from build123d import *

# Parameters (mm, degrees)
SKETCH1_W              = 144.4879
SKETCH1_H              = 47.625
SKETCH1_R              = 14.3129
BOSS_EXTRUDE1_DEPTH    = 6.35
FILLET1_R              = 6.35
F_10_32_TAPPED_HOLE1_D = 4.0386
F_10_32_TAPPED_HOLE2_D = 4.0386
CUT_EXTRUDE1_DEPTH     = 147.5745916
FILLET2_R              = 2.54


with BuildPart() as part:
    # Sketch1 → Boss-Extrude1 (new body)
    with BuildSketch(Plane(origin=(0, 0, 0), x_dir=(0, 0, -1), z_dir=(1, 0, 0))):
        with Locations((-72.24395, 0)):
            Rectangle(SKETCH1_W, SKETCH1_H)
        with Locations((-120.65, 0)):
            Circle(SKETCH1_R, mode=Mode.SUBTRACT)
    extrude(amount=BOSS_EXTRUDE1_DEPTH)

    # Fillet1
    fillet1_edges = [part.edges().sort_by_distance(p)[0] for p in [
        (3.175, -23.8125, 144.4879),
        (3.175, 23.8125, 144.4879),
        (3.175, 23.8125, 0),
        (3.175, -23.8125, 0),
    ]]
    fillet(fillet1_edges, radius=FILLET1_R)

    # #10-32 Tapped Hole1 (through all)
    with Locations(Plane.ZY):
        with Locations((103.1875, 17.4625), (138.1125, 17.4625), (138.1125, -17.4625), (103.1875, -17.4625)):
            Hole(F_10_32_TAPPED_HOLE1_D / 2)

    # #10-32 Tapped Hole2 (through all)
    with Locations(Plane(origin=(6.35, 0, 0), x_dir=(0, 0, -1), z_dir=(1, 0, 0))):
        with Locations((-12.7, 14.2875), (-38.1, 14.2875), (-38.1, -11.1125), (-12.7, -11.1125)):
            Hole(F_10_32_TAPPED_HOLE2_D / 2)

    # Sketch8 → Cut-Extrude1 (cut, through all)
    with BuildSketch(Plane(origin=(6.35, 0, 0), x_dir=(0, 0, -1), z_dir=(1, 0, 0))):
        with BuildLine():
            Line((-80.436721657, 17.4625), (-53.975, 17.4625))
            ThreePointArc((-53.975, 17.4625), (-51.72993597, 16.53256403), (-50.8, 14.2875))
            Line((-50.8, 14.2875), (-50.8, -5.989274253))
            ThreePointArc((-50.8, -5.989274253), (-52.569784121, -8.836376874), (-55.906137534, -8.509459331))
            Line((-55.906137534, -8.509459331), (-82.367859191, 11.767314922))
            ThreePointArc((-82.367859191, 11.767314922), (-83.443564904, 15.307067893), (-80.436721657, 17.4625))
        make_face()
        with BuildLine():
            Line((-93.6625, 5.989274253), (-93.6625, -14.2875))
            ThreePointArc((-93.6625, -14.2875), (-92.73256403, -16.53256403), (-90.4875, -17.4625))
            Line((-90.4875, -17.4625), (-64.025778343, -17.4625))
            ThreePointArc((-64.025778343, -17.4625), (-61.018935096, -15.307067893), (-62.094640809, -11.767314922))
            Line((-62.094640809, -11.767314922), (-88.556362466, 8.509459331))
            ThreePointArc((-88.556362466, 8.509459331), (-91.892715879, 8.836376874), (-93.6625, 5.989274253))
        make_face()
        with BuildLine():
            Line((-38.1, 19.05), (-12.7, 19.05))
            ThreePointArc((-12.7, 19.05), (-16.728416874, 16.827827486), (-16.997532015, 12.235032015))
            Line((-16.997532015, 12.235032015), (-25.4, 3.83256403))
            Line((-25.4, 3.83256403), (-33.802467985, 12.235032015))
            ThreePointArc((-33.802467985, 12.235032015), (-34.071583126, 16.827827486), (-38.1, 19.05))
        make_face()
        with BuildLine():
            Line((-7.9375, 14.2875), (-7.9375, -11.1125))
            ThreePointArc((-7.9375, -11.1125), (-10.159672514, -7.084083126), (-14.752467985, -6.814967985))
            Line((-14.752467985, -6.814967985), (-23.15493597, 1.5875))
            Line((-23.15493597, 1.5875), (-14.752467985, 9.989967985))
            ThreePointArc((-14.752467985, 9.989967985), (-10.159672514, 10.259083126), (-7.9375, 14.2875))
        make_face()
        with BuildLine():
            Line((-38.1, -15.875), (-12.7, -15.875))
            ThreePointArc((-12.7, -15.875), (-16.728416874, -13.652827486), (-16.997532015, -9.060032015))
            Line((-16.997532015, -9.060032015), (-25.4, -0.65756403))
            Line((-25.4, -0.65756403), (-33.802467985, -9.060032015))
            ThreePointArc((-33.802467985, -9.060032015), (-34.071583126, -13.652827486), (-38.1, -15.875))
        make_face()
        with BuildLine():
            Line((-42.8625, 14.2875), (-42.8625, -11.1125))
            ThreePointArc((-42.8625, -11.1125), (-40.640327486, -7.084083126), (-36.047532015, -6.814967985))
            Line((-36.047532015, -6.814967985), (-27.64506403, 1.5875))
            Line((-27.64506403, 1.5875), (-36.047532015, 9.989967985))
            ThreePointArc((-36.047532015, 9.989967985), (-40.640327486, 10.259083126), (-42.8625, 14.2875))
        make_face()
    extrude(amount=-CUT_EXTRUDE1_DEPTH, mode=Mode.SUBTRACT)

    # Fillet2
    fillet2_edges = [part.edges().sort_by_distance(p)[0] for p in [
        (3.175, -15.875, 12.7),
    ]]
    fillet(fillet2_edges, radius=FILLET2_R)
    fillet2_2_edges = [part.edges().sort_by_distance(p)[0] for p in [
        (3.175, -9.060032015, 16.997532015),
    ]]
    fillet(fillet2_2_edges, radius=FILLET2_R)
    fillet2_3_edges = [part.edges().sort_by_distance(p)[0] for p in [
        (3.175, -0.65756403, 25.4),
    ]]
    fillet(fillet2_3_edges, radius=FILLET2_R)
    fillet2_4_edges = [part.edges().sort_by_distance(p)[0] for p in [
        (3.175, -9.060032015, 33.802467985),
    ]]
    fillet(fillet2_4_edges, radius=FILLET2_R)
    fillet2_5_edges = [part.edges().sort_by_distance(p)[0] for p in [
        (3.175, 14.2875, 42.8625),
    ]]
    fillet(fillet2_5_edges, radius=FILLET2_R)
    fillet2_6_edges = [part.edges().sort_by_distance(p)[0] for p in [
        (3.175, -6.814967985, 36.047532015),
    ]]
    fillet(fillet2_6_edges, radius=FILLET2_R)
    fillet2_7_edges = [part.edges().sort_by_distance(p)[0] for p in [
        (3.175, 1.5875, 27.64506403),
    ]]
    fillet(fillet2_7_edges, radius=FILLET2_R)
    fillet2_8_edges = [part.edges().sort_by_distance(p)[0] for p in [
        (3.175, 9.989967985, 36.047532015),
    ]]
    fillet(fillet2_8_edges, radius=FILLET2_R)
    fillet2_9_edges = [part.edges().sort_by_distance(p)[0] for p in [
        (3.175, 14.2875, 7.9375),
    ]]
    fillet(fillet2_9_edges, radius=FILLET2_R)
    fillet2_10_edges = [part.edges().sort_by_distance(p)[0] for p in [
        (3.175, 9.989967985, 14.752467985),
    ]]
    fillet(fillet2_10_edges, radius=FILLET2_R)
    fillet2_11_edges = [part.edges().sort_by_distance(p)[0] for p in [
        (3.175, 1.5875, 23.15493597),
    ]]
    fillet(fillet2_11_edges, radius=FILLET2_R)
    fillet2_12_edges = [part.edges().sort_by_distance(p)[0] for p in [
        (3.175, -6.814967985, 14.752467985),
    ]]
    fillet(fillet2_12_edges, radius=FILLET2_R)
    fillet2_13_edges = [part.edges().sort_by_distance(p)[0] for p in [
        (3.175, -11.1125, 7.9375),
    ]]
    fillet(fillet2_13_edges, radius=FILLET2_R)
    fillet2_14_edges = [part.edges().sort_by_distance(p)[0] for p in [
        (3.175, 19.05, 38.1),
    ]]
    fillet(fillet2_14_edges, radius=FILLET2_R)
    fillet2_15_edges = [part.edges().sort_by_distance(p)[0] for p in [
        (3.175, 12.235032015, 33.802467985),
    ]]
    fillet(fillet2_15_edges, radius=FILLET2_R)
    fillet2_16_edges = [part.edges().sort_by_distance(p)[0] for p in [
        (3.175, 3.83256403, 25.4),
    ]]
    fillet(fillet2_16_edges, radius=FILLET2_R)
    fillet2_17_edges = [part.edges().sort_by_distance(p)[0] for p in [
        (3.175, 12.235032015, 16.997532015),
    ]]
    fillet(fillet2_17_edges, radius=FILLET2_R)
    fillet2_18_edges = [part.edges().sort_by_distance(p)[0] for p in [
        (3.175, 19.05, 12.7),
    ]]
    fillet(fillet2_18_edges, radius=FILLET2_R)
    fillet2_19_edges = [part.edges().sort_by_distance(p)[0] for p in [
        (3.175, -15.875, 38.1),
    ]]
    fillet(fillet2_19_edges, radius=FILLET2_R)
    fillet2_20_edges = [part.edges().sort_by_distance(p)[0] for p in [
        (3.175, -11.1125, 42.8625),
    ]]
    fillet(fillet2_20_edges, radius=FILLET2_R)


solid = part.part
Could you check a few things on this model? Use its own coordinates, in mm. A direction names the side the tool comes from. Round coordinates to 2 decimals unless told otherwise and drop trailing zeros. Write each loop counter-clockwise with the first axis right and the second up, starting at its lowest first coordinate (ties: lowest second). Pieces come first, ordered by that corner, then holes. Notation, with made-up numbers: (88.25, 6) - (101.25, 6) arc R20 ccw to (101.25, 43) - close; hole circle Ø6 at (-35, 76). An arc over 180 degrees is marked (long way). Put each result on its own line as item: value. Start each with the question number.
(1) I want a section at B-B, the plane z = 74. Please give me the cut outline in (x, y), plus the area to 3 significant figures.
(2) Will this pin go through, and if not, where does the flat tip stop? pin 1 (5.5 mm diameter, centred on y = 14.29, z = 12.7, fed in from -X).
(3) I want a section at D-D, the plane z = 59. Please give me the cut outline in (x, y).
(4) For faces 1 (the flat face through (3, -23.812, 73)), 2 (the cylindrical face through (3.131, -14.86, 17.625)), which set-ups out of +Z, -Z, +X, -X, +Y, -Y let a thin tool reach every point of the face, with its end or its side?
(5) I need wall thicknesses on probe 1 along Z at (x, y) = (2, 3); probe 2 along Z at (x, y) = (2.5, -19); probe 3 along Y at (x, z) = (0.5, 63.5). Which ranges of each line are inside material? Lowest first, please.
(6) I want a section at A-A, the plane z = 120.65. Please give me the cut outline in (x, y).
(7) Thinking about a two-plate mould opening in Z: for faces 3 (the cylindrical face through (3.2, -8.8, 52.5)), 4 (the cylindrical face through (3.131, -6.188, 41.847)), 5 (the flat face through (0, 0, 73)), 6 (the cylindrical face through (3.22, -22, 1.91)), which applies, released by +Z, released by -Z, zero draft, split by the parting line, or undercut?
(8) I want a section at C-C, the plane x = 2.75. Give the number of separate pieces and of enclosed holes in the cut face, plus the area to 3 significant figures.
Here are the results:
1. outline: (0, -23.81) - (6.35, -23.81) - (6.35, -17.46) - (0, -17.46) - close; (0, -2.64) - (6.35, -2.64) - (6.35, 5.36) - (0, 5.36) - close; (0, 17.46) - (6.35, 17.46) - (6.35, 23.81) - (0, 23.81) - close
1. area: 131 mm^2
2. pin 1: stops at x = 0
3. outline: (0, -23.81) - (6.35, -23.81) - (6.35, -6.14) - (0, -6.14) - close; (0, 17.46) - (6.35, 17.46) - (6.35, 23.81) - (0, 23.81) - close
4. face 1: +Z, -Z, +X, -X, -Y
4. face 2: +X, -X
5. probe 1: z = 0 to 7.94, 21.67 to 29.13, 42.86 to 50.8, 70.93 to 81.37, 93.66 to 106.66, 134.64 to 144.49
5. probe 2: z = 0.19 to 101.88, 104.5 to 136.8, 139.42 to 144.3
5. probe 3: y = -23.81 to -17.42, -10.69 to -2.69, 17.46 to 23.81
6. outline: (0, -23.81) - (6.35, -23.81) - (6.35, -14.31) - (0, -14.31) - close; (0, 14.31) - (6.35, 14.31) - (6.35, 23.81) - (0, 23.81) - close
7. face 3: undercut
7. face 4: undercut
7. face 5: zero draft
7. face 6: released by -Z
8. separate pieces: 1
8. enclosed holes: 15
8. area: 4,280 mm^2
